Verification items for this drawing (mm, ordinates from the low corner). Round coordinates to 2 decimals unless told otherwise and drop trailing zeros. Order: outer loops, then holes, each group sorted by start corner. A loop starts at its lowest first (then second) coordinate and runs counter-clockwise, first axis right, second up. Notation, with made-up numbers: M 28,68.5 L 51,68.5 A7 ccw 51,77.5 Z; hole C -39.75,21.5 d11. An arc over 180 degrees is marked long. Use CSV: the item, a comma, the result in double quotes. Start each with the question number.
Q1. Gauge pin test, flat ends, axial feed: pin 1 Ø1.5 at (x, z) = (18.5, 26) entering from -Y; pin 2 Ø3 at (y, z) = (28.5, 11) entering from -X; pin 3 Ø2 at (x, y) = (25, 25) entering from -Z; pin 4 Ø2 at (y, z) = (29, 10.5) entering from +X. Record the tip position at first contact, or that the pin passes through.
Q2. Sectioned sample at D-D (y = 12.25). Enter the section's corners in (x, z).
Q3. Mould release check, pull along Y, two halves, no side actions. Record for the marked faces 1, 2, 3 and 4: +Y half, -Y half, draft (parallel to the pull), parting line (faces both ways), or undercut.
Q4. Sectioned sample at A-A (z = 19). Enter the section's corners in (x, y), and give its area (3 significant figures).
Q5. Scan lines: line 1 (Y direction, x = 45.9, z = 28.75); line 2 (Y direction, x = 21, z = 19); line 3 (Z direction, x = 35, y = 18.75). Record each from-to range of solid material in increasing order.
Q6. Sectioned sample at C-C (y = 25). Enter the section's corners in (x, z).
Q7. Sectioned sample at B-B (x = 45.9). Enter the section's corners in (y, z), and give its area (3 significant figures).
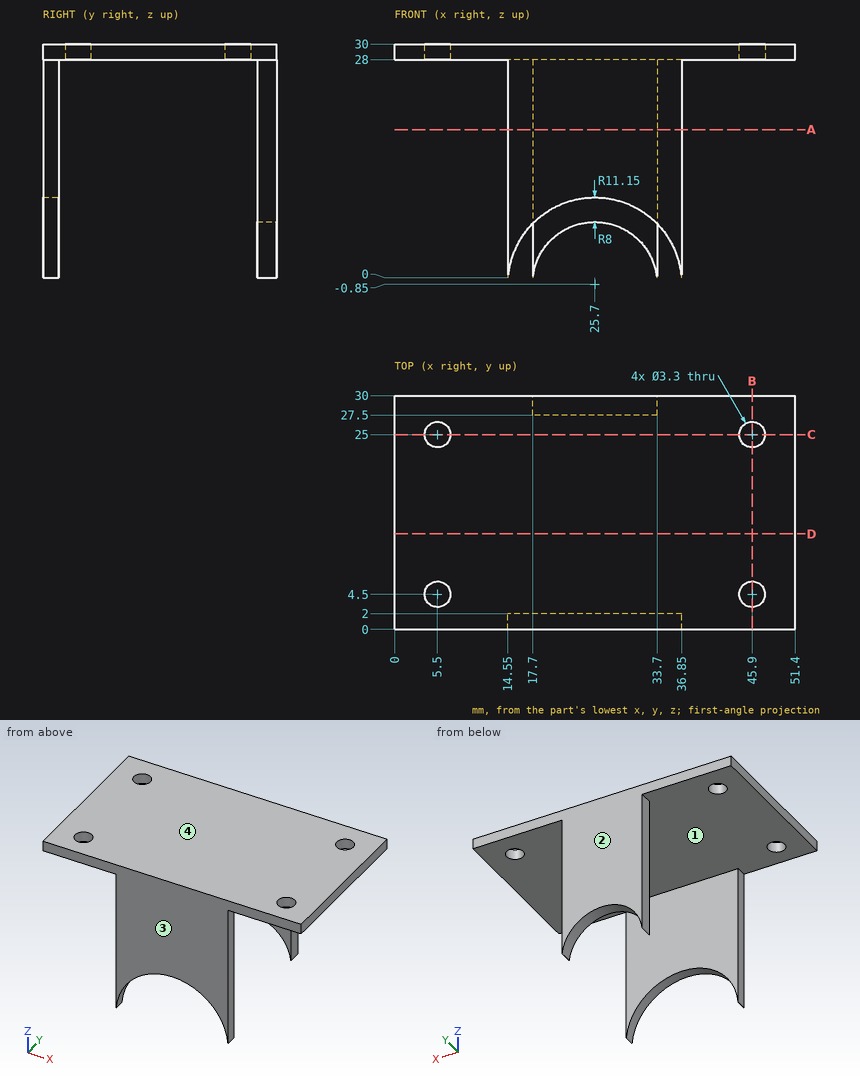
Verdict:
1,pin 1,"stops at y = 0"
1,pin 2,"stops at x = 17.7"
1,pin 3,"stops at z = 28"
1,pin 4,"stops at x = 33.7"
2,outline,"M 0,28 L 51.4,28 L 51.4,30 L 0,30 Z"
3,face 1,"undercut"
3,face 2,"+Y half"
3,face 3,"-Y half"
3,face 4,"draft"
4,outline,"M 14.55,0 L 36.85,0 L 36.85,2 L 14.55,2 Z; M 17.7,27.5 L 33.7,27.5 L 33.7,30 L 17.7,30 Z"
4,area,"84.6 mm²"
5,line 1,"y = 0 to 2.85, 6.15 to 23.35, 26.65 to 30"
5,line 2,"y = 0 to 2, 27.5 to 30"
5,line 3,"z = 28 to 30"
6,outline,"M 0,28 L 3.85,28 L 3.85,30 L 0,30 Z; M 7.15,28 L 44.25,28 L 44.25,30 L 7.15,30 Z; M 47.55,28 L 51.4,28 L 51.4,30 L 47.55,30 Z"
7,outline,"M 0,28 L 2.85,28 L 2.85,30 L 0,30 Z; M 6.15,28 L 23.35,28 L 23.35,30 L 6.15,30 Z; M 26.65,28 L 30,28 L 30,30 L 26.65,30 Z"
7,area,"46.8 mm²"
